Build history of the part. All positions in model axes, mm. Face numbers are marked on the shaded views. A direction names the side the tool comes from. Round coordinates to 2 decimals unless told otherwise and drop trailing zeros. Write each loop counter-clockwise with the first axis right and the second up, starting at its lowest first coordinate (ties: lowest second). Pieces come first, ordered by that corner, then holes. Notation, with made-up numbers: M -20,81 L 26,81 A11 ccw 26,94 Z; hole C -2.75,37 d7. An arc over 180 degrees is marked long. Write item = value, one per line. Start each with the question number.
Q1. Band-saw the part on C-C on y = 9. Write the cut outline in (x, z).
Q2. Band-saw the part on B-B on y = 13. Write the cut outline in (x, z).
Q3. Probe L1, parallel to X at y = 2.05, z = -5; L2, parallel to X at y = 10.5, z = -5; L3, parallel to Z at x = 5, y = 12.25. List the from-to ranges inside material, lowest first.
Q4. Band-saw the part on A-A on z = -5. Write the cut outline in (x, y), plus the area to 3 significant figures.
Q5. Pull direction X, two halves, no side cores. Call the marked faces 3, 4 and 5: released by +X, released by -X, zero draft, split by the parting line, or undercut.
Q6. Band-saw the part on D-D on x = 38. Write the cut outline in (y, z), plus the area to 3 significant figures.
Q7. Tool access for the marked faces 1 and 2: list every direction of +Z, -Z, +X, -X, +Y, -Y with a clear straight run to the whole face (end or side of a thin tool).
Q8. Drop flat-ended pins along their axis: P1, Ø5, axis at x = 18, z = -4.5, coming from the +Y side; P2, Ø5, axis at y = 4, z = -2.5, coming from the +X side; P3, Ø6, axis at x = 40.5, y = 9, coming from the -Z side. Give the stop position or say it passes through.
```python
from build123d import *

# Parameters (mm, degrees)
ESQUISSE1_R             = 2.65
BOSS_EXTRU_1_DEPTH      = 15
ESQUISSE2_R             = 3.488871883
ESQUISSE2_R_2           = 3.573781448
BOSS_EXTRU_2_DEPTH      = 4
ENL_V_START             = -5
ENL_V_MAT_EXTRU_1_DEPTH = 5
ESQUISSE8_R             = 2.65
BOSS_EXTRU_3_DEPTH      = 3


with BuildPart() as part:
    # Esquisse1 → Boss.-Extru.1 (new body)
    with BuildSketch(Plane(origin=(0, 0, 0), x_dir=(1, 0, 0), z_dir=(0, 1, 0))):
        with BuildLine():
            Line((5, 0), (34, 0))
            ThreePointArc((34, 0), (39, 5), (34, 10))
            Line((34, 10), (5, 10))
            ThreePointArc((5, 10), (0, 5), (5, 0))
        make_face()
        with Locations(Location((5, 5, 0), (0, 0, 270))):
            Circle(ESQUISSE1_R, mode=Mode.SUBTRACT)
        with Locations(Location((34, 5, 0), (0, 0, 270))):
            Circle(ESQUISSE1_R, mode=Mode.SUBTRACT)
    extrude(amount=BOSS_EXTRU_1_DEPTH)

    # Esquisse2 → Boss.-Extru.2 (add)
    with BuildSketch(Plane.XZ):
        with Locations((5, -5)):
            Circle(ESQUISSE2_R)
        with Locations((34, -5)):
            Circle(ESQUISSE2_R_2)
    extrude(amount=-BOSS_EXTRU_2_DEPTH)

    # Esquisse3 → Enlèv. mat.-Extru.1 (cut)
    with BuildSketch(Plane(origin=(0, 15, 0), x_dir=(1, 0, 0), z_dir=(0, 1, 0)).offset(ENL_V_START)):
        with BuildLine():
            Line((5, 10), (34, 10))
            ThreePointArc((34, 10), (29, 5), (34, 0))
            Line((34, 0), (5, 0))
            ThreePointArc((5, 0), (10, 5), (5, 10))
        make_face()
    extrude(amount=ENL_V_MAT_EXTRU_1_DEPTH, mode=Mode.SUBTRACT)

    # Esquisse8 → Boss.-Extru.3 (add)
    with BuildSketch(Plane.XZ):
        with BuildLine():
            Line((44.001861421, -10), (-5.001861421, -10))
            ThreePointArc((-5.001861421, -10), (-10.001861421, -5), (-5.001861421, 0))
            Line((-5.001861421, 0), (44.001861421, 0))
            ThreePointArc((44.001861421, 0), (49.001861421, -5), (44.001861421, -10))
        make_face()
        with Locations(Location((-5.001861421, -5, 0), (0, 0, 270))):
            Circle(ESQUISSE8_R, mode=Mode.SUBTRACT)
        with Locations(Location((44.001861421, -5, 0), (0, 0, 270))):
            Circle(ESQUISSE8_R, mode=Mode.SUBTRACT)
    extrude(amount=-BOSS_EXTRU_3_DEPTH)


solid = part.part
```
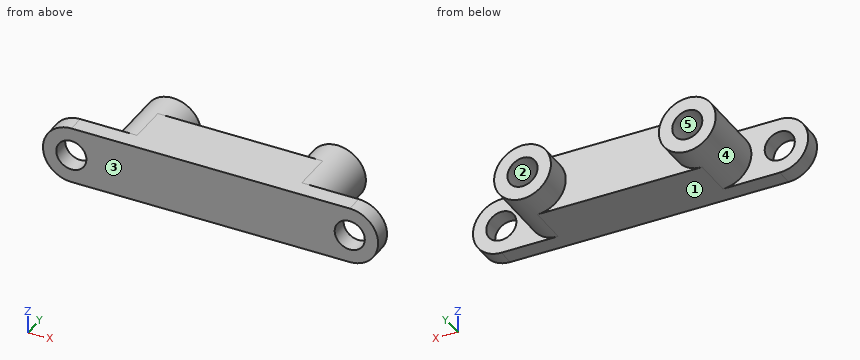
Conclusion:
q1.outline = M 5,-10 L 34,-10 A5 ccw 34,0 L 5,0 A5 ccw Z; hole C 5,-5 d5.3; hole C 34,-5 d5.3
q2.outline = C 5,-5 d10; C 34,-5 d10; hole C 5,-5 d5.3; hole C 34,-5 d5.3
q3.L1 = -10 to -7.65, -2.35 to 41.35, 46.65 to 49
q3.L2 = 0 to 2.35, 7.65 to 10, 29 to 31.35, 36.65 to 39
q3.L3 = -10 to -7.65, -2.35 to 0
q4.outline = M -10,0 L -7.65,0 L -7.65,3 L -10,3 Z; M -2.35,0 L 41.35,0 L 41.35,3 L 39,3 L 39,15 L 36.65,15 L 36.65,4 L 31.35,4 L 31.35,15 L 29,15 L 29,10 L 10,10 L 10,15 L 7.65,15 L 7.65,4 L 2.35,4 L 2.35,15 L 0,15 L 0,3 L -2.35,3 Z; M 46.65,0 L 49,0 L 49,3 L 46.65,3 Z
q4.area = 402 mm^2
q5.face_3 = zero draft
q5.face_4 = undercut
q5.face_5 = undercut
q6.outline = M 0,-10 L 3,-10 L 3,-8 L 15,-8 L 15,-2 L 3,-2 L 3,0 L 0,0 Z
q6.area = 102 mm^2
q7.face_1 = -Z, +X, -X, +Y, -Y
q7.face_2 = +Y
q8.P1 = 10
q8.P2 = 49
q8.P3 = -8.57
